Verification items for the finished model (mm, model axes). Face numbers are marked on the shaded views. Give positions to 0.01 mm unless a question says otherwise; leave off trailing zeros. Order: outer loops, then holes, each group sorted by start corner. A loop starts at its lowest first (then second) coordinate and runs counter-clockwise, first axis right, second up.
(1) Sectioned sample at C-C on x = 100. Record the cut outline in (y, z).
(2) Mould release check, pull along Y, two halves, no side actions. Record for the marked faces 1 and 2: pulls with the +Y half, pulls with the -Y half, needs draft (parallel to the pull), parting line crosses it, or undercut.
(3) Scan lines: L1, parallel to Z at x = -94, y = -11.25; L2, parallel to X at y = -10, z = 59; L3, parallel to X at y = -2.25, z = -167. Record each from-to range of solid material in increasing order.
(4) Sectioned sample at B-B on z = 0. Record the cut outline in (x, y).
(5) Sectioned sample at A-A on y = -6.25. Record the cut outline in (x, z).
(6) Gauge pin test, flat ends, axial feed: pin 1 (2 mm diameter, centred on x = 95, y = -5.5, fed in from +Z); pin 2 (4 mm diameter, centred on y = -11, z = 89, fed in from +X); pin 3 (3 mm diameter, centred on y = -6, z = 24.5, fed in from +X). Record the tip position at first contact, or that the pin passes through.
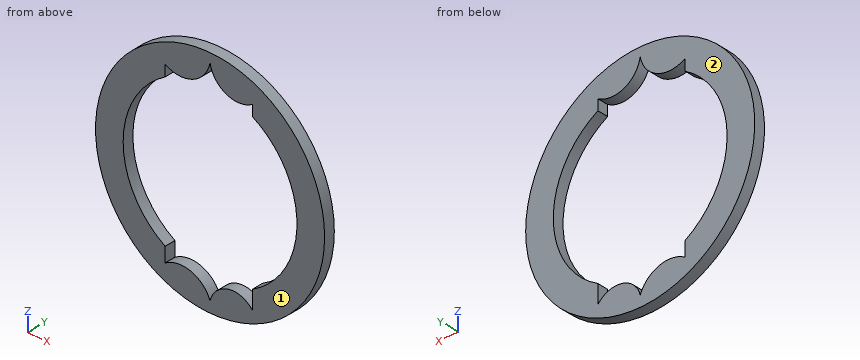
```python
from build123d import *

# Parameters (mm, degrees)
F0_R     = 192.393498
F1_DEPTH = 18.29249


with BuildPart() as f1:
    # F0 (on Front) → F1 (new body)
    with BuildSketch(Plane.XZ):
        Circle(F0_R)
        with BuildLine():
            ThreePointArc((-75.423603, -124.989932), (-145.983571, 0), (-75.423603, 124.989932))
            Line((-75.423603, 124.989932), (-75.423603, 143.759063))
            ThreePointArc((-75.423603, 143.759063), (-28.813946, 140.830175), (0, 177.583337))
            ThreePointArc((0, 177.583337), (26.867171, 142.388247), (71.053845, 145.230274))
            Line((71.053845, 145.230274), (71.053845, 127.52472))
            ThreePointArc((71.053845, 127.52472), (145.983571, 0), (71.053845, -127.52472))
            Line((71.053845, -127.52472), (71.053845, -150.177163))
            Line((71.053845, -150.177163), (71.053845, -158.453529))
            ThreePointArc((71.053845, -158.453529), (30.748142, -144.186111), (0, -173.895717))
            ThreePointArc((0, -173.895717), (-31.937801, -143.816001), (-75.423603, -149.629557))
            Line((-75.423603, -149.629557), (-75.423603, -124.989932))
        make_face(mode=Mode.SUBTRACT)
    extrude(amount=F1_DEPTH)


solid = f1.part
```
Ans:
1. outline: (-18.29, -164.36) - (0, -164.36) - (0, -106.35) - (-18.29, -106.35) - close; (-18.29, 106.35) - (0, 106.35) - (0, 164.36) - (-18.29, 164.36) - close
2. face 1: pulls with the -Y half
2. face 2: pulls with the +Y half
3. L1: z = -167.87 to -111.69, 111.69 to 167.87
3. L2: x = -183.12 to -133.53, 133.53 to 183.12
3. L3: x = -95.53 to -3.3, 2.43 to 95.53
4. outline: (-192.39, -18.29) - (-145.98, -18.29) - (-145.98, 0) - (-192.39, 0) - close; (145.98, -18.29) - (192.39, -18.29) - (192.39, 0) - (145.98, 0) - close
5. outline: circle Ø384.79 at (0, 0); hole (-75.42, -149.63) arc R51.05 cw to (0, -173.9) arc R40.62 cw to (71.05, -158.45) - (71.05, -127.52) arc R145.98 ccw to (71.05, 127.52) - (71.05, 145.23) arc R46.91 cw to (0, 177.58) arc R50.15 cw to (-75.42, 143.76) - (-75.42, 124.99) arc R145.98 ccw to (-75.42, -124.99) - close
6. pin 1: stops at z = 167.87
6. pin 2: stops at x = 171.6
6. pin 3: stops at x = 191.01
